Part model, mm, in its own coordinate system. A direction names the side the tool comes from. Round coordinates to 2 decimals unless told otherwise and drop trailing zeros. Write each loop counter-clockwise with the first axis right and the second up, starting at its lowest first coordinate (ties: lowest second). Pieces come first, ordered by that corner, then holes. Notation, with made-up numbers: (7, -7.5) -> (53, -7.5) arc R27 cw to (53, 18.5) -> close; hole circle Ø11 at (-27.75, -20.5). An arc over 180 degrees is marked (long way). Use CSV: the item, a comma, the result in double quotes. Start each with the question number.
(1) Saw through at B-B (z = -41). Give the cut face in (x, y) (3 decimals).
(2) Which spindle directions (+Z, -Z, +X, -X, +Y, -Y) get a long thin tool onto all of the face, cutting with end or side? Do faces 5 (the cylindrical face through (53.14, -55.004, -31.839)), 6 (the cylindrical face through (7.937, -69.92, -3.131)), 7 (the flat face through (59, -70, -6.35)). Say none if no direction does.
(3) Probe line 1 (X direction, y = 63, z = -17); line 2 (Y direction, x = -58, z = -7) (3 decimals); line 3 (X direction, y = -57, z = -27). List the from-to ranges inside material, lowest first. Write a range as [from, to].
(4) Saw through at D-D (x = 22.5). Give the cut face in (y, z) (3 decimals), plus the area to 3 significant figures.
(5) Saw through at C-C (y = 63.5). Give the cut face in (x, z).
(6) Drop flat-ended pins along their axis: pin 1 (3.5 mm diameter, centred on x = 28, y = -64.5, fed in from -Z); pin 2 (7.5 mm diameter, centred on x = -14, z = -26, fed in from -Y); pin 3 (4 mm diameter, centred on x = -4.5, z = -45, fed in from -Y). Give the stop position or say it passes through.
(7) Saw through at A-A (x = -31.75). Give the cut face in (y, z) (3 decimals), plus the area to 3 significant figures.
(8) Two-plate mould, pull along X, no slides. Class faces 1 (the flat face through (-1, 1, 0)), 2 (the flat face through (53.975, -70, -3)), 3 (the flat face through (0, -57, -25.4)), 4 (the flat face through (-63.5, 16, -25)): released by +X, released by -X, zero draft, split by the parting line, or undercut.
```python
from build123d import *

# Parameters (mm, degrees)
F0_W      = 127
F0_H      = 152.4
F1_DEPTH  = 50.8
F3_DEPTH  = 127.001
F5_DEPTH  = 12.7
F6_W      = 38.1
F6_H      = 6.35
F7_DEPTH  = 6.351
F8_R      = 6.35
F9_DEPTH  = 50.801
F11_DEPTH = 50.801


with BuildPart() as f1:
    # F0 (on Top) → F1 (new body)
    with BuildSketch(Plane.XY):
        Rectangle(F0_W, F0_H)
    extrude(amount=-F1_DEPTH)

    # F2 (on face) → F3 (cut, through all)
    with BuildSketch(Plane.YZ.offset(63.5)):
        Polygon((-76.2, -12.7), (-76.2, -50.8), (-50.8, -50.8), (-50.8, -38.1), (-63.5, -38.1), (-63.5, -12.7), (-66.675, -12.7), (-66.675, -6.35), (-73.025, -6.35), (-73.025, -12.7), align=None)
    extrude(amount=-F3_DEPTH, mode=Mode.SUBTRACT)

    # F4 (on face) → F5 (cut)
    with BuildSketch(Plane(origin=(0, 0, -38.1), x_dir=(1, 0, 0), z_dir=(0, 0, -1))):
        with BuildLine():
            ThreePointArc((-47.625, 57.15), (-50.8, 60.325), (-53.975, 57.15))
            Line((-53.975, 57.15), (-47.625, 57.15))
        make_face()
        with BuildLine():
            ThreePointArc((53.975, 57.15), (50.8, 60.325), (47.625, 57.15))
            Line((47.625, 57.15), (53.975, 57.15))
        make_face()
        with BuildLine():
            Line((53.975, 57.15), (47.625, 57.15))
            ThreePointArc((47.625, 57.15), (50.8, 53.975), (53.975, 57.15))
        make_face()
        with BuildLine():
            ThreePointArc((3.175, 57.15), (0, 60.325), (-3.175, 57.15))
            Line((-3.175, 57.15), (3.175, 57.15))
        make_face()
        with BuildLine():
            Line((3.175, 57.15), (-3.175, 57.15))
            ThreePointArc((-3.175, 57.15), (0, 53.975), (3.175, 57.15))
        make_face()
        with BuildLine():
            Line((-47.625, 57.15), (-53.975, 57.15))
            ThreePointArc((-53.975, 57.15), (-50.8, 53.975), (-47.625, 57.15))
        make_face()
    extrude(amount=-F5_DEPTH, mode=Mode.SUBTRACT)

    # F6 (on face) → F7 (cut, through all)
    with BuildSketch(Plane(origin=(0, 0, -6.35), x_dir=(1, 0, 0), z_dir=(0, 0, -1))):
        with Locations((-34.925, 69.85)):
            Rectangle(F6_W, F6_H)
        with Locations((34.925, 69.85)):
            Rectangle(F6_W, F6_H)
    extrude(amount=-F7_DEPTH, mode=Mode.SUBTRACT)

    # F8 (on face) → F9 (cut, through all)
    with BuildSketch(Plane.XY):
        with BuildLine():
            ThreePointArc((-38.1, 63.5), (-31.75, 57.15), (-25.4, 63.5))
            ThreePointArc((-25.4, 63.5), (-31.75, 69.85), (-38.1, 63.5))
        make_face()
        with BuildLine():
            ThreePointArc((-44.45, 47.625), (-45.379936, 49.870064), (-47.625, 50.8))
            ThreePointArc((-47.625, 50.8), (-49.870064, 45.379936), (-44.45, 47.625))
        make_face()
        with Locations((31.75, 63.5)):
            Circle(F8_R)
        with BuildLine():
            ThreePointArc((50.8, 47.625), (49.870064, 49.870064), (47.625, 50.8))
            ThreePointArc((47.625, 50.8), (45.379936, 45.379936), (50.8, 47.625))
        make_face()
    extrude(amount=-F9_DEPTH, mode=Mode.SUBTRACT)

    # F10 (on face) → F11 (cut, through all)
    with BuildSketch(Plane.XY):
        with BuildLine():
            Line((4.7625, -66.675), (-4.7625, -66.675))
            ThreePointArc((-4.7625, -66.675), (-7.9375, -69.85), (-4.7625, -73.025))
            Line((-4.7625, -73.025), (4.7625, -73.025))
            ThreePointArc((4.7625, -73.025), (7.9375, -69.85), (4.7625, -66.675))
        make_face()
    extrude(amount=-F11_DEPTH, mode=Mode.SUBTRACT)


solid = f1.part
```
Answers:
1,outline,"(-63.5, -50.8) -> (63.5, -50.8) -> (63.5, 76.2) -> (-63.5, 76.2) -> close; hole circle Ø6.35 at (-47.625, 47.625); hole circle Ø12.7 at (-31.75, 63.5); hole circle Ø12.7 at (31.75, 63.5); hole circle Ø6.35 at (47.625, 47.625)"
2,face 5,"-Z"
2,face 6,"+Z, -Z"
2,face 7,"-Z, +X, -X"
3,line 1,"x = [-63.5, -38.08], [-25.42, 25.42], [38.08, 63.5]"
3,line 2,"y = [-76.2, -73.025], [-66.675, 76.2]"
3,line 3,"x = [-63.5, -53.97], [-47.63, -3.17], [3.17, 47.63], [53.97, 63.5]"
4,outline,"(-76.2, -12.7) -> (-73.025, -12.7) -> (-73.025, 0) -> (-76.2, 0) -> close; (-66.675, -12.7) -> (-63.5, -12.7) -> (-63.5, -38.1) -> (-50.8, -38.1) -> (-50.8, -50.8) -> (76.2, -50.8) -> (76.2, 0) -> (-66.675, 0) -> close"
4,area,"7,020 mm²"
5,outline,"(-63.5, -50.8) -> (-38.1, -50.8) -> (-38.1, 0) -> (-63.5, 0) -> close; (-25.4, -50.8) -> (25.4, -50.8) -> (25.4, 0) -> (-25.4, 0) -> close; (38.1, -50.8) -> (63.5, -50.8) -> (63.5, 0) -> (38.1, 0) -> close"
6,pin 1,"stops at z = -38.1"
6,pin 2,"stops at y = -63.5"
6,pin 3,"stops at y = -50.8"
7,outline,"(-76.2, -12.7) -> (-73.025, -12.7) -> (-73.025, 0) -> (-76.2, 0) -> close; (-66.675, -12.7) -> (-63.5, -12.7) -> (-63.5, -38.1) -> (-50.8, -38.1) -> (-50.8, -50.8) -> (57.15, -50.8) -> (57.15, 0) -> (-66.675, 0) -> close; (69.85, -50.8) -> (76.2, -50.8) -> (76.2, 0) -> (69.85, 0) -> close"
7,area,"6,370 mm²"
8,face 1,"zero draft"
8,face 2,"undercut"
8,face 3,"undercut"
8,face 4,"released by -X"
